```python
from build123d import *

# Parameters (mm, degrees)
F1_DEPTH = 185.7375
F3_DEPTH = 76.2
F4_R     = 5.08


with BuildPart() as f1:
    # F0 (on Front) → F1 (new body, symmetric)
    with BuildSketch(Plane.XZ):
        Polygon((0, 76.2), (0, 0), (76.2, 0), (76.2, 9.525), (9.525, 9.525), (9.525, 76.2), align=None)
    extrude(amount=F1_DEPTH, both=True)

    # F2 (on face) → F3 (cut)
    with BuildSketch(Plane(origin=(0, 0, 0), x_dir=(0, -1, 0), z_dir=(-1, 0, 0))):
        Polygon((-185.7375, 76.2), (-185.7375, 0), (-118.558163, 76.2), align=None)
        Polygon((118.558163, 76.2), (185.7375, 0), (185.7375, 76.2), align=None)
    extrude(amount=-F3_DEPTH, mode=Mode.SUBTRACT)

    # F4
    f4_edges = [f1.edges().sort_by_distance(p)[0] for p in [
        (9.525, 0, 76.2),
        (9.525, 0, 9.525),
        (76.2, 0, 9.525),
    ]]
    fillet(f4_edges, radius=F4_R)


solid = f1.part
```
Can you work these out from the model? Positions are in its coordinate system, mm. A direction names the side the tool comes from. Round coordinates to 2 decimals unless told otherwise and drop trailing zeros. Loops run counter-clockwise (first coordinate to the right, second up) from the corner with the lowest first, then second, coordinate; pieces in that order, holes last.
Item 1: Which directions (+Z, -Z, +X, -X, +Y, -Y) give clear straight access to the entire face, cutting with the end or side of a thin tool? Please do faces 1 (the flat face through (9.525, -2, 42)), 2 (the flat face through (0, -3, 39)).
Item 2: Will these pins go through, and if not, where does the flat tip stop? pin 1 Ø17 at (x, y) = (29, 37) entering from +Z (3 decimals); pin 2 Ø12 at (x, z) = (18.5, 29) entering from -Y; pin 3 Ø3 at (y, z) = (-71.5, 14) entering from +X; pin 4 Ø1 at (y, z) = (-68.5, 9) entering from +X.
Item 3: Suppose I cut it at B-B, the plane z = 25.5. Write out the boundary of the cut face in (x, y) (3 decimals).
Item 4: Suppose I cut it at C-C, the plane x = 56. Write out the boundary of the cut face in (y, z) (1 decimal).
Item 5: Suppose I cut it at A-A, the plane y = -3. Write out the boundary of the cut face in (x, z) (3 decimals).
Item 6: Please list where these lines run through material, in increasing order: L1, parallel to Z at x = 69.5, y = 81.5 (3 decimals); L2, parallel to X at y = -36.5, z = 73.5.
Reported:
1. face 1: +Z, +X, +Y, -Y
1. face 2: +Z, -Z, -X, +Y, -Y
2. pin 1: stops at z = 9.525
2. pin 2: passes through
2. pin 3: stops at x = 9.98
2. pin 4: stops at x = 74.18
3. outline: (0, -163.256) - (9.525, -163.256) - (9.525, 163.256) - (0, 163.256) - close
4. outline: (-185.7, 0) - (185.7, 0) - (177.3, 9.5) - (-177.3, 9.5) - close
5. outline: (0, 0) - (76.2, 0) - (76.2, 4.445) arc R5.08 ccw to (71.12, 9.525) - (14.605, 9.525) arc R5.08 cw to (9.525, 14.605) - (9.525, 71.12) arc R5.08 ccw to (4.445, 76.2) - (0, 76.2) - close
6. L1: z = 0 to 9.525
6. L2: x = 0 to 8.93
